from build123d import *

# Parameters (mm, degrees)
F1_DEPTH = 1.5875


with BuildPart() as f1:
    # F0 (on Right) → F1 (new body)
    with BuildSketch(Plane.YZ):
        with BuildLine():
            ThreePointArc((0, -6.35), (4.4901280605, -4.4901280605), (6.35, 0))
            ThreePointArc((6.35, 0), (4.4901280605, 4.4901280605), (0, 6.35))
            Line((0, 6.35), (0, 3.175))
            ThreePointArc((0, 3.175), (2.2450640303, 2.2450640303), (3.175, 0))
            ThreePointArc((3.175, 0), (2.2450640303, -2.2450640303), (0, -3.175))
            Line((0, -3.175), (0, -6.35))
        make_face()
        with BuildLine():
            Line((0, 3.175), (0, 6.35))
            ThreePointArc((0, 6.35), (-6.35, 0), (0, -6.35))
            Line((0, -6.35), (0, -3.175))
            ThreePointArc((0, -3.175), (-3.175, 0), (0, 3.175))
        make_face()
        with BuildLine():
            ThreePointArc((0, -6.35), (-6.35, 0), (0, 6.35))
            Line((0, 6.35), (-22.225, 6.35))
            Line((-22.225, 6.35), (-22.225, -6.35))
            Line((-22.225, -6.35), (0, -6.35))
        make_face()
        with BuildLine():
            ThreePointArc((-9.525, -2.38125), (-8.9637339924, -2.6137339924), (-8.73125, -3.175))
            ThreePointArc((-8.73125, -3.175), (-8.9637339924, -3.7362660076), (-9.525, -3.96875))
            Line((-9.525, -3.96875), (-19.05, -3.96875))
            ThreePointArc((-19.05, -3.96875), (-19.84375, -3.175), (-19.05, -2.38125))
            Line((-19.05, -2.38125), (-9.525, -2.38125))
        make_face(mode=Mode.SUBTRACT)
        with BuildLine():
            ThreePointArc((-19.05, 2.38125), (-19.84375, 3.175), (-19.05, 3.96875))
            Line((-19.05, 3.96875), (-9.525, 3.96875))
            ThreePointArc((-9.525, 3.96875), (-8.9637339924, 3.7362660076), (-8.73125, 3.175))
            ThreePointArc((-8.73125, 3.175), (-8.9637339924, 2.6137339924), (-9.525, 2.38125))
            Line((-9.525, 2.38125), (-19.05, 2.38125))
        make_face(mode=Mode.SUBTRACT)
    extrude(amount=-F1_DEPTH)


solid = f1.part
Input: part model. Units: mm. Frame: model coordinates. A direction names the side the tool comes from. Coordinates: 2 decimals unless noted, no trailing zeros. Loops run counter-clockwise (first coordinate to the right, second up) from the corner with the lowest first, then second, coordinate; pieces in that order, holes last.
(1) Material intervals for probe 1 along Z at (x, y) = (-0.1, -11.75); probe 2 along Y at (x, z) = (-1.2, 2.5) (3 decimals), sorted ascending.
(2) Set-up query: faces 1 (the face through (-1, -22.225, 0)), 2 (the face through (-1, -14, 2.381)). Return all of +Z, -Z, +X, -X, +Y, -Y with unobstructed straight access to the full face (end or side cutting, diameter ignored); none if empty.
(3) Section C-C on z = 2. Return the cut outline in (x, y) (1 decimal).
(4) Section B-B on y = -14.25. Return the cut outline in (x, z), then the cut area to 3 significant figures.
(5) Section D-D on z = 5.5. Return the cut outline in (x, y) (1 decimal).
(6) Section A-A on x = -0.8. Count the separate pieces of the cut face and the enclosed holes in it, then the cut area to 3 significant figures.
(7) Pull-direction query (Z, two-part tool) for faces 3 (the face through (-1.588, -8, 0)), 4 (the face through (-1, -14, 3.969)), 5 (the face through (-1, -11, -6.35)); classes: released by +Z, released by -Z, zero draft, split by the parting line, or undercut.
Data:
1. probe 1: z = -6.35 to -3.97, -2.38 to 2.38, 3.97 to 6.35
1. probe 2: y = -22.225 to -19.468, -9.107 to -1.957, 1.957 to 5.837
2. face 1: +Z, -Z, +X, -X, -Y
2. face 2: +X, -X
3. outline: (-1.6, -22.2) - (0, -22.2) - (0, -2.5) - (-1.6, -2.5) - close; (-1.6, 2.5) - (0, 2.5) - (0, 6) - (-1.6, 6) - close
4. outline: (-1.59, -6.35) - (0, -6.35) - (0, -3.97) - (-1.59, -3.97) - close; (-1.59, -2.38) - (0, -2.38) - (0, 2.38) - (-1.59, 2.38) - close; (-1.59, 3.97) - (0, 3.97) - (0, 6.35) - (-1.59, 6.35) - close
4. area: 15.1 mm2
5. outline: (-1.6, -22.2) - (0, -22.2) - (0, 3.2) - (-1.6, 3.2) - close
6. separate pieces: 1
6. enclosed holes: 3
6. area: 280 mm2
7. face 3: zero draft
7. face 4: undercut
7. face 5: released by -Z
